Verification items for the finished model (mm, model axes). A direction names the side the tool comes from. Coordinates: 2 decimals unless noted, no trailing zeros. Order: outer loops, then holes, each group sorted by start corner. A loop starts at its lowest first (then second) coordinate and runs counter-clockwise, first axis right, second up. Notation, with made-up numbers: (20.5, 25) -> (62.5, 25) arc R17 cw to (62.5, 42) -> close; hole circle Ø10 at (19, 32). An arc over 180 degrees is marked (long way). Write item = value, one per line. Start each with the question number.
1. Cross-section at B-B on x = 57. Record the cut outline in (y, z).
2. Cross-section at A-A on y = 4.25. Record the cut outline in (x, z), plus the area to 3 significant figures.
3. Set-up check for faces 1 (the flat face through (0, 5, 7)), 2 (the flat face through (55, 3, 17)): record each of +Z, -Z, +X, -X, +Y, -Y from which the full face is reachable in a straight line by a thin tool's end or side.
4. Thickness scan on line 1 along X through (y, z) = (5.5, 9.5); line 2 along Z through (x, y) = (52.5, 4.25); line 3 along Y through (x, z) = (96.5, 6.75). Record the ranges inside material, lowest first. Write a range as from..to.
5. Cross-section at C-C on z = 8.75. Record the cut outline in (x, y), plus the area to 3 significant figures.
6. Release check for a two-part mould opening along Z. For faces 3 (the flat face through (55, 3, -2)), 4 (the flat face through (55, 5, 0)), 5 (the flat face through (114, 3, 7)) record: +Z half, -Z half, draft (parallel to the pull), parting line (faces both ways), or undercut.
from build123d import *

# Parameters (mm, degrees)
SKETCH_1_W      = 112
SKETCH_1_H      = 15
EXTRUDE_1_DEPTH = 3
SKETCH_2_W      = 116
SKETCH_2_H      = 19
SKETCH_2_W_2    = 112
SKETCH_2_H_2    = 15
EXTRUDE_2_DEPTH = 7


with BuildPart() as part:
    # 草图1 → 凸台-拉伸1 (new body)
    with BuildSketch(Plane(origin=(0, 0, 0), x_dir=(1, 0, 0), z_dir=(0, 1, 0))):
        with Locations((56, -7.5)):
            Rectangle(SKETCH_1_W, SKETCH_1_H)
    extrude(amount=EXTRUDE_1_DEPTH)

    # 草图2 → 凸台-拉伸2 (add)
    with BuildSketch(Plane.XZ):
        with Locations((56, 7.5)):
            Rectangle(SKETCH_2_W, SKETCH_2_H)
        with Locations((56, 7.5)):
            Rectangle(SKETCH_2_W_2, SKETCH_2_H_2, mode=Mode.SUBTRACT)
    extrude(amount=-EXTRUDE_2_DEPTH)


solid = part.part
Worked out:
q1.outline = (0, -2) -> (7, -2) -> (7, 0) -> (3, 0) -> (3, 15) -> (7, 15) -> (7, 17) -> (0, 17) -> close
q2.outline = (-2, -2) -> (114, -2) -> (114, 17) -> (-2, 17) -> close; hole (0, 0) -> (112, 0) -> (112, 15) -> (0, 15) -> close
q2.area = 524 mm²
q3.face_1 = +Y
q3.face_2 = +Z, +X, -X, +Y, -Y
q4.line_1 = -2..0, 112..114
q4.line_2 = -2..0, 15..17
q4.line_3 = 0..3
q5.outline = (-2, 0) -> (114, 0) -> (114, 7) -> (112, 7) -> (112, 3) -> (0, 3) -> (0, 7) -> (-2, 7) -> close
q5.area = 364 mm²
q6.face_3 = -Z half
q6.face_4 = undercut
q6.face_5 = draft
